```python
from build123d import *

# Parameters (mm, degrees)
SCHIZZO1_W                                   = 64.6
SCHIZZO1_H                                   = 20
ESTRUSIONE_ESTRUSIONE1_DEPTH                 = 8.2
SCHIZZO2_W                                   = 8.2
SCHIZZO2_H                                   = 20
ESTRUSIONE_ESTRUSIONE2_DEPTH                 = 28.9
SCHIZZO3_W                                   = 8.2
SCHIZZO3_H                                   = 20
ESTRUSIONE_ESTRUSIONE3_DEPTH                 = 28.9
SCHIZZO4_W                                   = 8.2
SCHIZZO4_H                                   = 20
ESTRUSIONE_ESTRUSIONE4_DEPTH                 = 8.2
SCHIZZO5_W                                   = 37.1
SCHIZZO5_H                                   = 20
ESTRUSIONE_ESTRUSIONE5_DEPTH                 = 8.2
SCHIZZO6_W                                   = 48.2
SCHIZZO6_H                                   = 20.7
TAGLIO_ESTRUSIONE1_DEPTH                     = 78.133455776
F_4_0_4_DIAMETER_HOLE2_D                     = 4
F_4_0_4_DIAMETER_HOLE2_DEPTH                 = 8.2
RACCORDO3_R                                  = 6
CBORE_FOR_M3_HEX_HEAD_CAP_SCREW1_D           = 3
CBORE_FOR_M3_HEX_HEAD_CAP_SCREW1_CBORE_D     = 7
CBORE_FOR_M3_HEX_HEAD_CAP_SCREW1_CBORE_DEPTH = 3
SKETCH5_W                                    = 46.4
SKETCH5_H                                    = 37.1
BOSS_EXTRUDE1_DEPTH                          = 10
FILLET3_R                                    = 6
CHAMFER2_SIZE                                = 10
CUT_EXTRUDE2_DEPTH                           = 2
SKETCH9_W                                    = 40.4
SKETCH9_H                                    = 8
BOSS_EXTRUDE2_DEPTH                          = 46.2
CBORE_FOR_M3_HEX_HEAD_CAP_SCREW2_D           = 3
CBORE_FOR_M3_HEX_HEAD_CAP_SCREW2_CBORE_D     = 7
CBORE_FOR_M3_HEX_HEAD_CAP_SCREW2_CBORE_DEPTH = 3
CUT_EXTRUDE3_DEPTH                           = 108.684957167
FILLET4_R                                    = 6
SKETCH15_W                                   = 8.2
SKETCH15_H                                   = 20
CUT_EXTRUDE4_DEPTH                           = 0.25
SKETCH16_W                                   = 8.2
SKETCH16_H                                   = 22
CUT_EXTRUDE5_DEPTH                           = 0.25
CUT_EXTRUDE6_DEPTH                           = 2
CUT_EXTRUDE7_DEPTH                           = 2
FILLET5_R                                    = 6
FILLET6_R                                    = 6


with BuildPart() as part:
    # Schizzo1 → Estrusione-Estrusione1 (new body)
    with BuildSketch(Plane.XY):
        with Locations((32.3, 10)):
            Rectangle(SCHIZZO1_W, SCHIZZO1_H)
    extrude(amount=ESTRUSIONE_ESTRUSIONE1_DEPTH)

    # Schizzo2 → Estrusione-Estrusione2 (add)
    with BuildSketch(Plane.XY.offset(8.2)):
        with Locations((4.1, 10)):
            Rectangle(SCHIZZO2_W, SCHIZZO2_H)
    extrude(amount=ESTRUSIONE_ESTRUSIONE2_DEPTH)

    # Schizzo3 → Estrusione-Estrusione3 (add)
    with BuildSketch(Plane.XY.offset(8.2)):
        with Locations((60.5, 10)):
            Rectangle(SCHIZZO3_W, SCHIZZO3_H)
    extrude(amount=ESTRUSIONE_ESTRUSIONE3_DEPTH)

    # Schizzo4 → Estrusione-Estrusione4 (add)
    with BuildSketch(Plane.ZY.offset(-56.4)):
        with Locations((33, 10)):
            Rectangle(SCHIZZO4_W, SCHIZZO4_H)
    extrude(amount=ESTRUSIONE_ESTRUSIONE4_DEPTH)

    # Schizzo5 → Estrusione-Estrusione5 (add)
    with BuildSketch(Plane.ZY):
        with Locations((18.55, 10)):
            Rectangle(SCHIZZO5_W, SCHIZZO5_H)
    extrude(amount=ESTRUSIONE_ESTRUSIONE5_DEPTH)

    # Schizzo6 → Taglio-Estrusione1 (cut, through all)
    with BuildSketch(Plane.XZ):
        with Locations((24.1, 18.55)):
            Rectangle(SCHIZZO6_W, SCHIZZO6_H)
    extrude(amount=-TAGLIO_ESTRUSIONE1_DEPTH, mode=Mode.SUBTRACT)

    # Ø4.0 (4) Diameter Hole2
    with Locations(Plane.XY.offset(37.1)):
        with Locations((51.7, 5), (4.7, 5), (4.7, 15), (51.7, 15)):
            Hole(F_4_0_4_DIAMETER_HOLE2_D / 2, depth=F_4_0_4_DIAMETER_HOLE2_DEPTH)

    # Raccordo3
    raccordo3_edges = [part.edges().sort_by_distance(p)[0] for p in [
        (64.6, 10, 37.1),
        (64.6, 10, 0),
    ]]
    fillet(raccordo3_edges, radius=RACCORDO3_R)

    # CBORE for M3 Hex Head Cap Screw1 (through all)
    with Locations(Plane.XY.offset(8.2)):
        with Locations((36.4, 10), (12.4, 10)):
            CounterBoreHole(CBORE_FOR_M3_HEX_HEAD_CAP_SCREW1_D / 2, CBORE_FOR_M3_HEX_HEAD_CAP_SCREW1_CBORE_D / 2, CBORE_FOR_M3_HEX_HEAD_CAP_SCREW1_CBORE_DEPTH)

    # Sketch5 → Boss-Extrude1 (add)
    with BuildSketch(Plane(origin=(0, 20, 0), x_dir=(1, 0, 0), z_dir=(0, 1, 0))):
        with Locations((15, -18.55)):
            Rectangle(SKETCH5_W, SKETCH5_H)
    extrude(amount=BOSS_EXTRUDE1_DEPTH)

    # Fillet3
    fillet3_edges = [part.edges().sort_by_distance(p)[0] for p in [
        (-8.2, 15, 37.1),
        (-8.2, 15, 0),
    ]]
    fillet(fillet3_edges, radius=FILLET3_R)

    # Chamfer2
    chamfer2_edges = [part.edges().sort_by_distance(p)[0] for p in [
        (38.2, 20, 4.1),
    ]]
    chamfer(chamfer2_edges, length=CHAMFER2_SIZE - 0.0001)  # a hair under: the kernel refuses the full size

    # Sketch8 → Cut-Extrude2 (cut)
    with BuildSketch(Plane(origin=(0, 20, 0), x_dir=(-1, 0, 0), z_dir=(0, -1, 0))):
        Polygon((-38.2, -37.1), (-38.2, -8.2), (0, -8.2), (0, -28.9), (-8.2, -28.9), (-8.2, -37.1), align=None)
    extrude(amount=-CUT_EXTRUDE2_DEPTH, mode=Mode.SUBTRACT)

    # Sketch9 → Boss-Extrude2 (add)
    with BuildSketch(Plane.XY.offset(37.1)):
        with Locations((18, 26)):
            Rectangle(SKETCH9_W, SKETCH9_H)
    extrude(amount=BOSS_EXTRUDE2_DEPTH)

    # CBORE for M3 Hex Head Cap Screw2 (through all)
    with Locations(Plane(origin=(0, 22, 0), x_dir=(-1, 0, 0), z_dir=(0, -1, 0))):
        with Locations((-22.6, -41.7), (-32.1, -41.7), (-22.6, -75.7), (-32.1, -75.7)):
            CounterBoreHole(CBORE_FOR_M3_HEX_HEAD_CAP_SCREW2_D / 2, CBORE_FOR_M3_HEX_HEAD_CAP_SCREW2_CBORE_D / 2, CBORE_FOR_M3_HEX_HEAD_CAP_SCREW2_CBORE_DEPTH)

    # Sketch13 → Cut-Extrude3 (cut, through all)
    with BuildSketch(Plane(origin=(0, 22, 0), x_dir=(-1, 0, 0), z_dir=(0, -1, 0))):
        Polygon((-16.6, -75.7), (-16.6, -83.3), (2.2, -83.3), (2.2, -37.1), align=None)
    extrude(amount=-CUT_EXTRUDE3_DEPTH, mode=Mode.SUBTRACT)

    # Fillet4
    fillet4_edges = [part.edges().sort_by_distance(p)[0] for p in [
        (38.2, 26, 83.3),
    ]]
    fillet(fillet4_edges, radius=FILLET4_R)

    # Sketch15 → Cut-Extrude4 (cut)
    with BuildSketch(Plane.ZY.offset(-48.2)):
        with Locations((33, 10)):
            Rectangle(SKETCH15_W, SKETCH15_H)
    extrude(amount=-CUT_EXTRUDE4_DEPTH, mode=Mode.SUBTRACT)

    # Sketch16 → Cut-Extrude5 (cut)
    with BuildSketch(Plane(origin=(8.2, 0, 0), x_dir=(0, 0, -1), z_dir=(1, 0, 0))):
        with Locations((-33, 11)):
            Rectangle(SKETCH16_W, SKETCH16_H)
    extrude(amount=-CUT_EXTRUDE5_DEPTH, mode=Mode.SUBTRACT)

    # Sketch21 → Cut-Extrude6 (cut)
    with BuildSketch(Plane(origin=(0, 30, 0), x_dir=(1, 0, 0), z_dir=(0, 1, 0))):
        Polygon((-2.2, -37.1), (16.6, -37.1), (16.6, -75.7), align=None)
    extrude(amount=-CUT_EXTRUDE6_DEPTH, mode=Mode.SUBTRACT)

    # Sketch22 → Cut-Extrude7 (cut)
    with BuildSketch(Plane(origin=(0, 22, 0), x_dir=(-1, 0, 0), z_dir=(0, -1, 0))):
        Polygon((2.2, -37.1), (-16.6, -37.1), (-16.6, -75.7), align=None)
    extrude(amount=-CUT_EXTRUDE7_DEPTH, mode=Mode.SUBTRACT)

    # Fillet5
    fillet5_edges = [part.edges().sort_by_distance(p)[0] for p in [
        (16.6, 26, 83.3),
    ]]
    fillet(fillet5_edges, radius=FILLET5_R)

    # Fillet6
    fillet6_edges = [part.edges().sort_by_distance(p)[0] for p in [
        (16.6, 29, 37.1),
        (16.6, 23, 37.1),
    ]]
    fillet(fillet6_edges, radius=FILLET6_R)


solid = part.part
```
The listing builds one solid part. Answer for the finished solid, in the listing's coordinates (mm). A direction names the side the tool comes from. Coordinates: 2 decimals unless noted, no trailing zeros. Loops run counter-clockwise (first coordinate to the right, second up) from the corner with the lowest first, then second, coordinate; pieces in that order, holes last. Notation, with made-up numbers: M 18.25,19.25 L 69.25,19.25 A14 ccw 69.25,35.25 Z; hole C 72,-25.5 d9. An arc over 180 degrees is marked long. Answer as a JSON object with one key per item and string values. Group by question number.
Item 1: Section B-B (y = 5) is taken. Write down the section's boundary in (x, z), and give its area (3 significant figures).
Item 2: Each of these flat-tipped pins is pushed along its axis until it touches: P1, Ø5.5, axis at x = 11.5, z = 64.5, coming from the -Y side; P2, Ø6.5, axis at y = 25.5, z = 35, coming from the +X side; P3, Ø11, axis at x = 51, y = 9.5, coming from the +Z side. Where does it stop, or does it pass through?
Item 3: Section C-C (z = 20.5) is taken. Write down the section's boundary in (x, y), and give its area (3 significant figures).
Item 4: Which of the six approach directions +Z, -Z, +X, -X, +Y, -Y give full straight-line access (tool end or side, diameter ignored) to faces 1 (the face through (23.359, 23.479, 45.117)), 2 (the face through (14.889, 28.986, 38.904)), 3 (the face through (48.45, 10, 33)), 4 (the face through (56.4, 10, 18)), 5 (the face through (3, 12, 37.1))?
Item 5: Section D-D (x = 4.7) is taken. Write down the section's boundary in (y, z), and give its area (3 significant figures).
Item 6: Determine the mould class of faces 6 (the face through (31, 25, 77)), 7 (the face through (39.633, 8.659, 6.721)), 8 (the face through (37.6, 9.1, 2.6)), 9 (the face through (30.485, 23.479, 44.805)) for opening direction Y: +Y half, -Y half, draft (parallel to the pull), parting line (faces both ways), or undercut.
Item 7: Section A-A (z = 36) is taken. Write down the section's boundary in (x, y).
Item 8: Consider L1, parallel to Z at x = 32.1, y = 26.45; L2, parallel to X at y = 27.9, z = 75.7; L3, parallel to X at y = 22.95, z = 75.7. Determine where each line is inside the solid, lowest interval first.
Solved:
{
 "1": {"outline": "M -8.2,6 A6 ccw -2.2,0 L 58.6,0 A6 ccw 64.6,6 L 64.6,31.1 A6 ccw 58.6,37.1 L 53.7,37.1 L 53.7,28.9 L 56.4,28.9 L 56.4,8.2 L 0,8.2 L 0,28.9 L 2.7,28.9 L 2.7,37.1 L -2.2,37.1 A6 ccw -8.2,31.1 Z; M 6.7,28.9 L 7.95,28.9 L 7.95,37.1 L 6.7,37.1 Z; M 48.45,28.9 L 49.7,28.9 L 49.7,37.1 L 48.45,37.1 Z", "area": "1,100 mm2"},
 "2": {"P1": "stops at y = 24", "P2": "stops at x = 38.2", "P3": "stops at z = 37.1"},
 "3": {"outline": "M -8.2,0 L 0,0 L 0,22 L 38.2,22 L 38.2,30 L -8.2,30 Z; M 56.4,0 L 64.6,0 L 64.6,20 L 56.4,20 Z", "area": "716 mm2"},
 "4": {"face 1": "-Y", "face 2": "+Z, -X, +Y", "face 3": "+Z, +Y, -Y", "face 4": "+Y, -Y", "face 5": "+Z, -X, -Y"},
 "5": {"outline": "M 0,0 L 30,0 L 30,37.1 L 28,37.1 L 28,51.27 L 24,51.27 L 24,37.1 L 17,37.1 L 17,28.9 L 22,28.9 L 22,8.2 L 0,8.2 Z; M 0,28.9 L 3,28.9 L 3,37.1 L 0,37.1 Z; M 7,28.9 L 13,28.9 L 13,37.1 L 7,37.1 Z", "area": "649 mm2"},
 "6": {"face 6": "-Y half", "face 7": "undercut", "face 8": "undercut", "face 9": "draft"},
 "7": {"outline": "M -5.66,0 L 7.95,0 L 7.95,22 L 38.2,22 L 38.2,30 L -5.66,30 Z; M 48.45,0 L 62.06,0 L 62.06,20 L 48.45,20 Z; hole C 4.7,5 d4; hole C 4.7,15 d4; hole C 51.7,5 d4; hole C 51.7,15 d4"},
 "8": {"L1": "z = 0 to 40.2, 43.2 to 74.2, 77.2 to 83.3", "L2": "x = 16.6 to 21.1, 24.1 to 30.6, 33.6 to 38.2", "L3": "x = 16.6 to 19.1, 26.1 to 28.6, 35.6 to 38.2"}
}
